```python
from build123d import *

# Parameters (mm, degrees)
BOSS_EXTRUDE1_DEPTH = 3.175


with BuildPart() as part:
    # Sketch1 → Boss-Extrude1 (new body)
    with BuildSketch(Plane(origin=(0, 0, 0), x_dir=(1, 0, 0), z_dir=(0, 1, 0))):
        with BuildLine():
            Line((-152.4, 0), (107.95, 0))
            Line((107.95, 0), (107.95, 38.1))
            Line((107.95, 38.1), (38.1, 101.6))
            Line((38.1, 101.6), (0, 101.6))
            add(Edge.make_bspline(
                [(-152.4, 38.1), (-93.526008547, 62.630829772), (-55.632677833, 62.244474427), (-13.235249882, 81.341283437), (-16.312722453, 94.803032311), (0, 101.6)],
                knots=[0, 0, 0, 0, 0.617418124, 0.717418124, 1, 1, 1, 1], degree=3))
            Line((-152.4, 38.1), (-152.4, 0))
        make_face()
    extrude(amount=BOSS_EXTRUDE1_DEPTH)


solid = part.part
```
Design review of the part built by this model. Coordinates are the model's own, in mm. Round coordinates to 2 decimals unless told otherwise and drop trailing zeros. Write each loop counter-clockwise with the first axis right and the second up, starting at its lowest first coordinate (ties: lowest second). Pieces come first, ordered by that corner, then holes.
Item 1: We need section A-A on x = 67. Write out the cut boundary in (y, z) (3 decimals), and give its area (3 significant figures).
Item 2: For probe 1 along Z at (x, y) = (-107.5, 1); probe 2 along Z at (x, y) = (48.5, 2.45); probe 3 along X at (y, z) = (1.85, -80.5), list the stretches that pass through material, from the lowest coordinate up.
Item 3: Clearance check with a flat-ended pin moving along its axis: pin 1 Ø1 at (x, y) = (-50, 1.5) entering from +Z. State where the tip first meets the part, or that it passes through.
Returned:
1. outline: (0, -75.327) - (3.175, -75.327) - (3.175, 0) - (0, 0) - close
1. area: 239 mm2
2. probe 1: z = -53.97 to 0
2. probe 2: z = -92.15 to 0
2. probe 3: x = -19.97 to 61.31
3. pin 1: stops at z = 0
